```python
from build123d import *

# Parameters (mm, degrees)
SKETCH1_R            = 7.5
BOSS_EXTRUDE1_DEPTH  = 3
M4_CLEARANCE_HOLE1_D = 4.3
SKETCH4_R            = 1
BOSS_EXTRUDE2_DEPTH  = 2


with BuildPart() as part:
    # Sketch1 → Boss-Extrude1 (new body)
    with BuildSketch(Plane(origin=(0, 0, 0), x_dir=(1, 0, 0), z_dir=(0, 1, 0))):
        with Locations(Location((0, 0, 0), (0, 0, 270))):
            Circle(SKETCH1_R)
    extrude(amount=BOSS_EXTRUDE1_DEPTH)

    # M4 Clearance Hole1 (through all)
    with Locations(Plane(origin=(0, 3, 0), x_dir=(1, 0, 0), z_dir=(0, 1, 0))):
        with Locations((0, 0)):
            Hole(M4_CLEARANCE_HOLE1_D / 2)

    # Sketch4 → Boss-Extrude2 (add)
    with BuildSketch(Plane.XZ):
        with Locations(Location((0, -5.5, 0), (0, 0, 90))):
            Circle(SKETCH4_R)
        with Locations(Location((4.763139721, 2.75, 0), (0, 0, 90))):
            Circle(SKETCH4_R)
        with Locations(Location((-4.763139721, 2.75, 0), (0, 0, 90))):
            Circle(SKETCH4_R)
    extrude(amount=BOSS_EXTRUDE2_DEPTH)


solid = part.part
```
Check sheet for the modelled part. Datum: model origin and axes. Units: mm. A direction names the side the tool comes from. Round coordinates to 2 decimals unless told otherwise and drop trailing zeros. Order: outer loops, then holes, each group sorted by start corner. A loop starts at its lowest first (then second) coordinate and runs counter-clockwise, first axis right, second up.
1) Go/stop test with flat-tipped pins: pin 1 Ø3 at (x, y) = (-5, -1) entering from -Z; pin 2 Ø1.5 at (x, y) = (-4.5, 2.5) entering from +Z. Record where each tip stops, or that it passes through.
2) Section check D-D (z = -5). Record the boundary of the cut face in (x, y).
3) Section check B-B (z = 0). Record the boundary of the cut face in (x, y).
4) Mould release check, pull along X, two halves, no side actions. Record for faces 1 (the cylindrical face through (2.15, 1.48, -0.09)), 2 (the cylindrical face through (0.33, 1.479, -7.493)), 3 (the flat face through (-2, 3, 2)): +X half, -X half, draft (parallel to the pull), parting line (faces both ways), or undercut.
5) Tool access check on faces 4 (the cylindrical face through (0.6, -1, -6.3)), 5 (the flat face through (5, -2, 3)). Record the directions out of +Z, -Z, +X, -X, +Y, -Y that give a thin tool (end or side, any length) a straight path to the whole face; none if there is none.
6) Section check C-C (y = 2.05). Record the boundary of the cut face in (x, z).
7) Scan lines: line 1 (Y direction, x = 2.25, z = 2.25); line 2 (X direction, y = -1.05, z = -5.5); line 3 (X direction, y = 1.9, z = -1.25). Record each from-to range of solid material in increasing order.
8) Section check A-A (x = 0). Record the boundary of the cut face in (y, z), and give its area (3 significant figures).
Result:
1. pin 1: stops at z = -6.42
1. pin 2: stops at z = 6.5
2. outline: (-5.59, 0) - (-0.87, 0) - (-0.87, -2) - (0.87, -2) - (0.87, 0) - (5.59, 0) - (5.59, 3) - (-5.59, 3) - close
3. outline: (-7.5, 0) - (-2.15, 0) - (-2.15, 3) - (-7.5, 3) - close; (2.15, 0) - (7.5, 0) - (7.5, 3) - (2.15, 3) - close
4. face 1: undercut
4. face 2: parting line
4. face 3: draft
5. face 4: -Y
5. face 5: +Z, -Z, +X, -X, -Y
6. outline: circle Ø15 at (0, 0); hole circle Ø4.3 at (0, 0)
7. line 1: y = 0 to 3
7. line 2: x = -1 to 1
7. line 3: x = -7.4 to -1.75, 1.75 to 7.4
8. outline: (-2, -6.5) - (0, -6.5) - (0, -7.5) - (3, -7.5) - (3, -2.15) - (0, -2.15) - (0, -4.5) - (-2, -4.5) - close; (0, 2.15) - (3, 2.15) - (3, 7.5) - (0, 7.5) - close
8. area: 36.1 mm2
